Design review of the part shown in the three views and the two pictorial views. Dimensions are in mm from the part's minimum x, y and z. Round coordinates to 2 decimals unless told otherwise and drop trailing zeros. Loops run counter-clockwise (first coordinate to the right, second up) from the corner with the lowest first, then second, coordinate; pieces in that order, holes last.
1) Take a section at B-B (z = 22). State the section outline as (x, y) points.
2) Insertion check: pin 1 (1 mm diameter, centred on x = 31.5, y = 5, fed in from +Z); pin 2 (1.8 mm diameter, centred on y = 3, z = 78.5, fed in from +X); pin 3 (1.8 mm diameter, centred on y = 3, z = 4.5, fed in from -X). Each pin has a flat end and moves straight along its axis. Give the tip position at first contact, or say it passes through.
3) Wall thickness on L1, parallel to Z at x = 145.5, y = 5.65; L2, parallel to X at y = 3.1, z = 52; L3, parallel to X at y = 5.35, z = 83.5: over which ranges is each line inside the solid? List them lowest first.
4) Take a section at C-C (x = 88). State the section outline as (y, z) points, then the cut area to 3 significant figures.
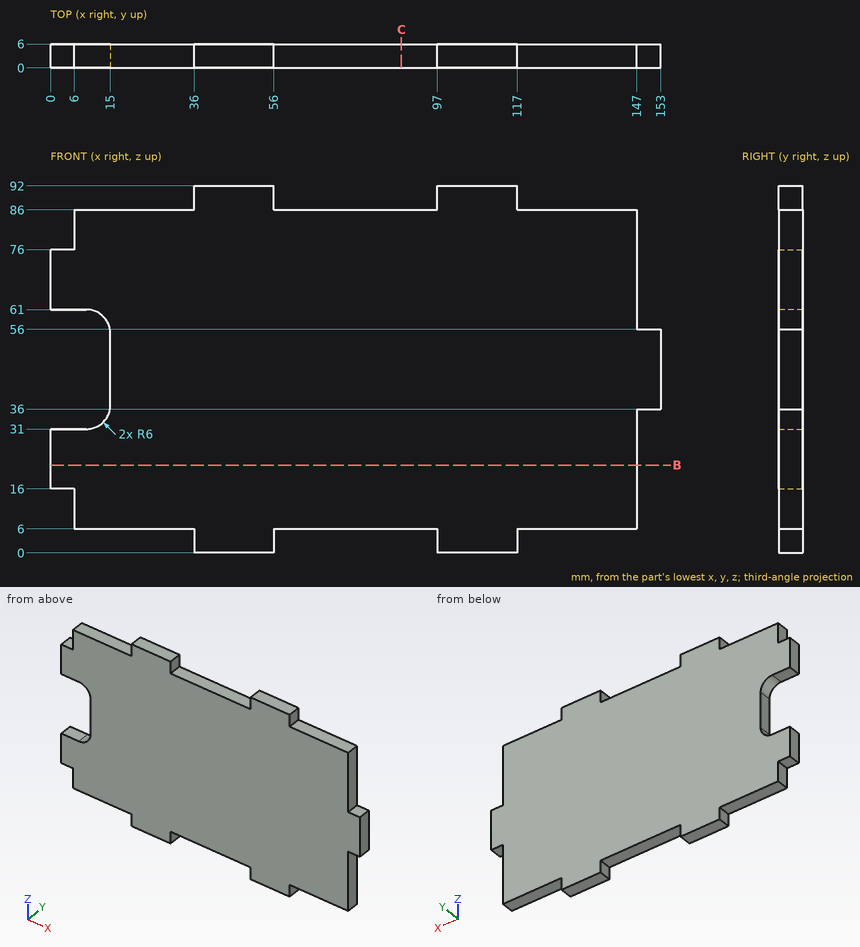
Response:
1. outline: (0, 0) - (147, 0) - (147, 6) - (0, 6) - close
2. pin 1: stops at z = 86
2. pin 2: stops at x = 147
2. pin 3: stops at x = 36
3. L1: z = 6 to 86
3. L2: x = 15 to 153
3. L3: x = 6 to 147
4. outline: (0, 6) - (6, 6) - (6, 86) - (0, 86) - close
4. area: 480 mm2
